Model file for the job. Use its own axes, mm. Face numbers are marked on the shaded views. A direction names the side the tool comes from. Coordinates: 2 decimals unless noted, no trailing zeros. Write each loop counter-clockwise with the first axis right and the second up, starting at its lowest first coordinate (ties: lowest second). Pieces come first, ordered by that corner, then holes.
Q1. Band-saw the part on D-D, the plane z = 33.5. Write the cut outline in (x, y).
Q2. Band-saw the part on A-A, the plane z = 20.5. Write the cut outline in (x, y), plus the area to 3 significant figures.
Q3. Band-saw the part on B-B, the plane x = -33. Write the cut outline in (y, z), plus the area to 3 significant figures.
Q4. Drill centre lines: probe 1 along X at (y, z) = (27, 29); probe 2 along Y at (x, z) = (5, -34); probe 3 along Z at (x, y) = (17, 21). Where is each one in solid material? Low to high.
Q5. Band-saw the part on C-C, the plane y = 23.5. Write the cut outline in (x, z), plus the area to 3 significant figures.
Q6. Which spindle directions (+Z, -Z, +X, -X, +Y, -Y) get a long thin tool onto all of the face, cutting with end or side? Do the marked faces 4, 5 and 6. Say none if no direction does.
Q7. Pull direction Y, two halves, no side cores. Call the marked faces 1, 2 and 3: released by +Y, released by -Y, zero draft, split by the parting line, or undercut.
Q8. Pin check, flat tips, straight feed: P1, Ø0.6, axis at y = 44, z = 29, coming from the -X side; P2, Ø12, axis at y = 13.5, z = -34, coming from the +X side; P3, Ø5, axis at y = 59.5, z = 10, coming from the -X side. Stop position of each tip, or through.
from build123d import *

# Parameters (mm, degrees)
SKETCH2_W           = 100
SKETCH2_H           = 100
BOSS_EXTRUDE1_DEPTH = 10
SKETCH3_W           = 75
SKETCH3_H           = 75
BOSS_EXTRUDE2_DEPTH = 10
SKETCH4_W           = 60
SKETCH4_H           = 60
BOSS_EXTRUDE3_DEPTH = 45
SKETCH5_W           = 80
SKETCH5_H           = 80
BOSS_EXTRUDE4_DEPTH = 10
FILLET2_R           = 10
FILLET1_R           = 10
FILLET3_R           = 10
SKETCH6_W           = 56
SKETCH6_H           = 31
CUT_EXTRUDE1_DEPTH  = 1.95
CIRPATTERN2_COUNT   = 4


# Some blends are built 0.0001 mm under size
with BuildPart() as part:
    # Sketch2 → Boss-Extrude1 (new body)
    with BuildSketch(Plane(origin=(0, 0, 0), x_dir=(1, 0, 0), z_dir=(0, 1, 0))):
        Rectangle(SKETCH2_W, SKETCH2_H)
    extrude(amount=BOSS_EXTRUDE1_DEPTH)

    # Sketch3 → Boss-Extrude2 (add)
    with BuildSketch(Plane(origin=(0, 10, 0), x_dir=(1, 0, 0), z_dir=(0, 1, 0))):
        Rectangle(SKETCH3_W, SKETCH3_H)
    extrude(amount=BOSS_EXTRUDE2_DEPTH)

    # Sketch4 → Boss-Extrude3 (add)
    with BuildSketch(Plane(origin=(0, 20, 0), x_dir=(1, 0, 0), z_dir=(0, 1, 0))):
        Rectangle(SKETCH4_W, SKETCH4_H)
    extrude(amount=BOSS_EXTRUDE3_DEPTH)

    # Sketch5 → Boss-Extrude4 (add)
    with BuildSketch(Plane(origin=(0, 65, 0), x_dir=(1, 0, 0), z_dir=(0, 1, 0))):
        Rectangle(SKETCH5_W, SKETCH5_H)
    extrude(amount=BOSS_EXTRUDE4_DEPTH)

    # Fillet2
    # the kernel refuses this fillet: 10 mm, written as the material it takes off along each edge
    with BuildSketch(Plane(origin=(-50, 10, 75), x_dir=(1, 0, 0), z_dir=(0, 0, -1)), Plane(origin=(75, 10, 50), x_dir=(0, 0, -1), z_dir=(-1, 0, 0)), Plane(origin=(-75, 10, -50), x_dir=(0, 0, 1), z_dir=(1, 0, 0)), Plane(origin=(50, 10, -75), x_dir=(-1, 0, 0), z_dir=(0, 0, 1))) as fillet2_piece_1:
        with BuildLine():
            CenterArc((FILLET2_R, FILLET2_R), FILLET2_R, 180, 90)
            Line((0, FILLET2_R), (-FILLET2_R * 0.02, FILLET2_R))
            Line((-FILLET2_R * 0.02, FILLET2_R), (-FILLET2_R * 0.02, -FILLET2_R * 0.02))
            Line((-FILLET2_R * 0.02, -FILLET2_R * 0.02), (FILLET2_R, -FILLET2_R * 0.02))
            Line((FILLET2_R, -FILLET2_R * 0.02), (FILLET2_R, 0))
        make_face()
    extrude(amount=150, mode=Mode.SUBTRACT)
    with BuildSketch(Plane(origin=(-37.5, 20, 61.706145914), x_dir=(1, 0, 0), z_dir=(0, 0, -1)), Plane(origin=(-61.706145914, 20, -37.5), x_dir=(0, 0, 1), z_dir=(1, 0, 0)), Plane(origin=(37.5, 20, -61.706145914), x_dir=(-1, 0, 0), z_dir=(0, 0, 1)), Plane(origin=(61.706145914, 20, 37.5), x_dir=(0, 0, -1), z_dir=(-1, 0, 0))) as fillet2_piece_2:
        with BuildLine():
            CenterArc((10, 9.682458366), FILLET2_R, 180, 75.522487814)
            Line((0, 9.682458366), (-0.2, 9.682458366))
            Line((-0.2, 9.682458366), (-0.2, 0))
            Line((-0.2, 0), (0, -0.2))
            ThreePointArc((0, -0.2), (3.75, -0.2), (7.45, -0.193649167))
            Line((7.45, -0.193649167), (7.5, 0))
        make_face()
    extrude(amount=123.412291828, mode=Mode.SUBTRACT)

    # Fillet1
    fillet1_edges = [part.edges().sort_by_distance(p)[0] for p in [
        (30, 65, 0),
        (0, 65, -30),
        (-30, 65, 0),
        (0, 65, 30),
    ]]
    fillet(fillet1_edges, radius=FILLET1_R - 0.0001)  # a hair under: the kernel refuses the full size

    # Fillet3
    # the kernel refuses this fillet: 10 mm, written as the material it takes off along each edge
    with BuildSketch(Plane(origin=(58.301375851, 65, 40), x_dir=(0, -0.25881282131019395, -0.9659274939277055), z_dir=(-1, 0, 0)), Plane(origin=(-40, 65, 58.301375851), x_dir=(0.9659274939277057, -0.2588128213101933, 0), z_dir=(0, 0, -1)), Plane(origin=(-58.301375851, 65, -40), x_dir=(0, -0.2588128213101933, 0.9659274939277057), z_dir=(1, 0, 0)), Plane(origin=(40, 65, -58.301375851), x_dir=(-0.9659274939277057, -0.2588128213101933, 0), z_dir=(0, 0, 1))) as fillet3_piece_1:
        with BuildLine():
            CenterArc((7.764622652, -9.659249058), FILLET3_R, 105.000203777, 60.000165399)
            Line((-1.894652287, -7.071120845), (-2.860579781, -6.812308023))
            Line((-2.860579781, -6.812308023), (-0.965927494, 0.258812821))
            Line((-0.965927494, 0.258812821), (0.258812821, 0.965927494))
            ThreePointArc((0.258812821, 0.965927494), (0.258909414, 0.965901613), (4.917575367, 0.965924906))
            Line((4.917575367, 0.965924906), (5.176397847, 0))
        make_face()
    extrude(amount=116.602751703, mode=Mode.SUBTRACT)

    # Sketch6 → Cut-Extrude1 (cut)
    with BuildSketch(Plane.XY.offset(30)):
        with Locations((0, 37.5)):
            Rectangle(SKETCH6_W, SKETCH6_H)
    cut_extrude1 = extrude(amount=-CUT_EXTRUDE1_DEPTH, mode=Mode.SUBTRACT)

    # CirPattern2: Cut-Extrude1 ×4 about axis
    cirpattern2_axis = Axis((0, 0, 0), (0, 1, 0))
    for i in range(1, CIRPATTERN2_COUNT):
        add(cut_extrude1.rotate(cirpattern2_axis, i * 360 / CIRPATTERN2_COUNT), mode=Mode.SUBTRACT)


solid = part.part
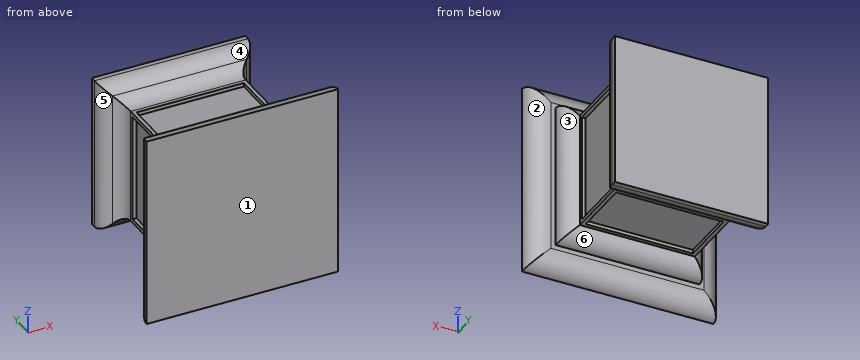
Answer sheet:
1. outline: (-50, 0) - (50, 0) arc R10 ccw to (40, 10) - (37.5, 10) - (37.5, 10.32) arc R10 ccw to (33.5, 18.32) - (-33.5, 18.32) arc R10 ccw to (-37.5, 10.32) - (-37.5, 10) - (-40, 10) arc R10 ccw to start; (-40, 72.32) arc R10 ccw to (-35, 63.66) arc R10 cw to (-33.5, 62.6) - (33.5, 62.6) arc R10 cw to (35, 63.66) arc R10 ccw to (40, 72.32) - (40, 75) - (-40, 75) - close
2. outline: (-50, 0) - (50, 0) arc R10 ccw to (40, 10) - (37.5, 10) - (37.5, 10.32) arc R10 ccw to (30, 20) - (30, 22) - (28.05, 22) - (28.05, 53) - (30, 53) - (30, 55) arc R10 cw to (35, 63.66) arc R10 ccw to (40, 72.32) - (40, 75) - (-40, 75) - (-40, 72.32) arc R10 ccw to (-35, 63.66) arc R10 cw to (-30, 55) - (-30, 53) - (-28.05, 53) - (-28.05, 22) - (-30, 22) - (-30, 20) arc R10 ccw to (-37.5, 10.32) - (-37.5, 10) - (-40, 10) arc R10 ccw to start
2. area: 5,080 mm2
3. outline: (0, -50) arc R10 ccw to (10, -40) - (10, -37.5) - (10.32, -37.5) arc R10 ccw to (18.67, -33) - (18.67, 33) arc R10 ccw to (10.32, 37.5) - (10, 37.5) - (10, 40) arc R10 ccw to (0, 50) - close; (62.14, -33) arc R10 cw to (63.66, -35) arc R10 ccw to (72.32, -40) - (75, -40) - (75, 40) - (72.32, 40) arc R10 ccw to (63.66, 35) arc R10 cw to (62.14, 33) - close
3. area: 2,570 mm2
4. probe 1: x = -30 to -28, 28 to 30
4. probe 2: y = 0 to 17.92, 63 to 75
4. probe 3: z = -30 to 30
5. outline: (-30, -30) - (-28, -30) - (-28, -28.05) - (28, -28.05) - (28, -30) - (30, -30) - (30, -28) - (28.05, -28) - (28.05, 28) - (30, 28) - (30, 30) - (28, 30) - (28, 28.05) - (-28, 28.05) - (-28, 30) - (-30, 30) - (-30, 28) - (-28.05, 28) - (-28.05, -28) - (-30, -28) - close
5. area: 3,160 mm2
6. face 4: +Z, +X, -X
6. face 5: +Z, -Z, -X
6. face 6: -Z, +X, -X
7. face 1: released by -Y
7. face 2: released by +Y
7. face 3: undercut
8. P1: stops at x = -30
8. P2: stops at x = 46.61
8. P3: stops at x = -32.86
